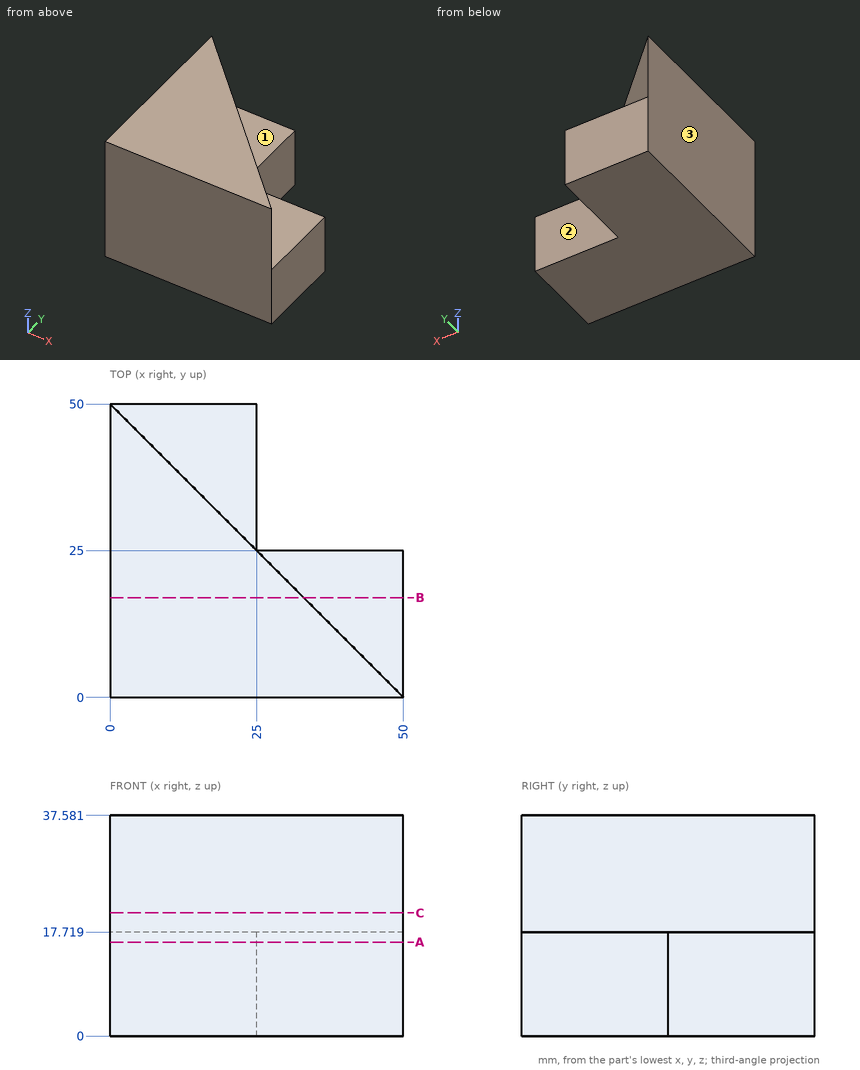
Answer from the drawing. Dimensions are ordinates in mm from the lowest x, y and z of the part. A direction names the side the tool comes from. Give positions to 0.01 mm unless a question says otherwise; leave off trailing zeros. Loops run counter-clockwise (first coordinate to the right, second up) from the corner with the lowest first, then second, coordinate; pieces in that order, holes last. Notation, with made-up numbers: (6, 30.5) -> (14, 30.5) arc R20 ccw to (14, 47.5) -> close; hole circle Ø11 at (-22.75, 15.25). An arc over 180 degrees is marked (long way). Answer as CSV lines item,"result".
Item 1: For the marked faces 1, 2 and 3, determine the directions among +Z, -Z, +X, -X, +Y, -Y from which every point of the face is accessible in a straight line to the end or side of a thin tool.
Returned:
face 1,"+Z, +X, +Y"
face 2,"+Z, -Z, +X, +Y"
face 3,"+Z, -Z, -X, +Y, -Y"
Item 2: Find section C-C on z = 21. Give the vertices of the cut face in (x, y).
Returned:
outline,"(0, 0) -> (50, 0) -> (0, 50) -> close"
Item 3: Find section A-A on z = 16. Give the vertices of the cut face in (x, y), plus the area to 4 significant figures.
Returned:
outline,"(0, 0) -> (50, 0) -> (50, 25) -> (25, 25) -> (25, 50) -> (0, 50) -> close"
area,"1,875 mm²"
Item 4: Find section B-B on y = 17. Give the vertices of the cut face in (x, z).
Returned:
outline,"(0, 0) -> (50, 0) -> (50, 17.72) -> (33, 17.72) -> (33, 37.58) -> (0, 37.58) -> close"
Item 5: Each of these flat-tipped pins is pushed along its axis until it touches: pin 1 (19.5 mm diameter, centred on x = 38, z = 6, fed in from +Y); pin 2 (8 mm diameter, centred on y = 32, z = 30, fed in from +X); pin 3 (14 mm diameter, centred on y = 40, z = 9, fed in from +X). Where does it stop, or does it pass through?
Returned:
pin 1,"stops at y = 25"
pin 2,"stops at x = 22"
pin 3,"stops at x = 25"
Item 6: Consider line 1 (Y direction, x = 33.5, z = 10.5); line 2 (Z direction, x = 24, y = 40.5). Determine where each line is inside the solid, lowest interval first. Write a range as [from, to].
Returned:
line 1,"y = [0, 25]"
line 2,"z = [0, 17.72]"
